Source: three-view drawing plus pictorial views. Frame: mm from the lowest corner of the part. Give positions to 0.01 mm unless a question says otherwise; leave off trailing zeros. Order: outer loops, then holes, each group sorted by start corner. A loop starts at its lowest first (then second) coordinate and runs counter-clockwise, first axis right, second up. Notation, with made-up numbers: (84.25, 56) - (120.25, 56) arc R23 ccw to (120.25, 79) - close; hole circle Ø10 at (39.5, 83). An arc over 180 degrees is marked (long way). Answer in a Markdown table with one row per item. Add a question column.
1. Ray query, line 1 (Z direction, x = 4, y = 61); line 2 (X direction, y = 32, z = 4.25). Return the intervals inside material, ascending. Write a range as [from, to].
2. Section query B-B on y = 40. Return loops of the section in (x, z).
3. Section query A-A on x = 4. Return loops of the section in (y, z), and give its area (3 significant figures).
4. Section query C-C on z = 1. Return loops of the section in (x, y).
5. Contact query for flat-ended pins moving along their axis: pin 1 (1.1 mm diameter, centred on y = 62, z = 7.5, fed in from -X); pin 2 (1 mm diameter, centred on x = 1.5, z = 5, fed in from -Y); pin 3 (0.8 mm diameter, centred on y = 2.5, z = 7.5, fed in from -X); pin 4 (0.8 mm diameter, centred on y = 3, z = 7.5, fed in from +X). Output: stop coordinate, or through.
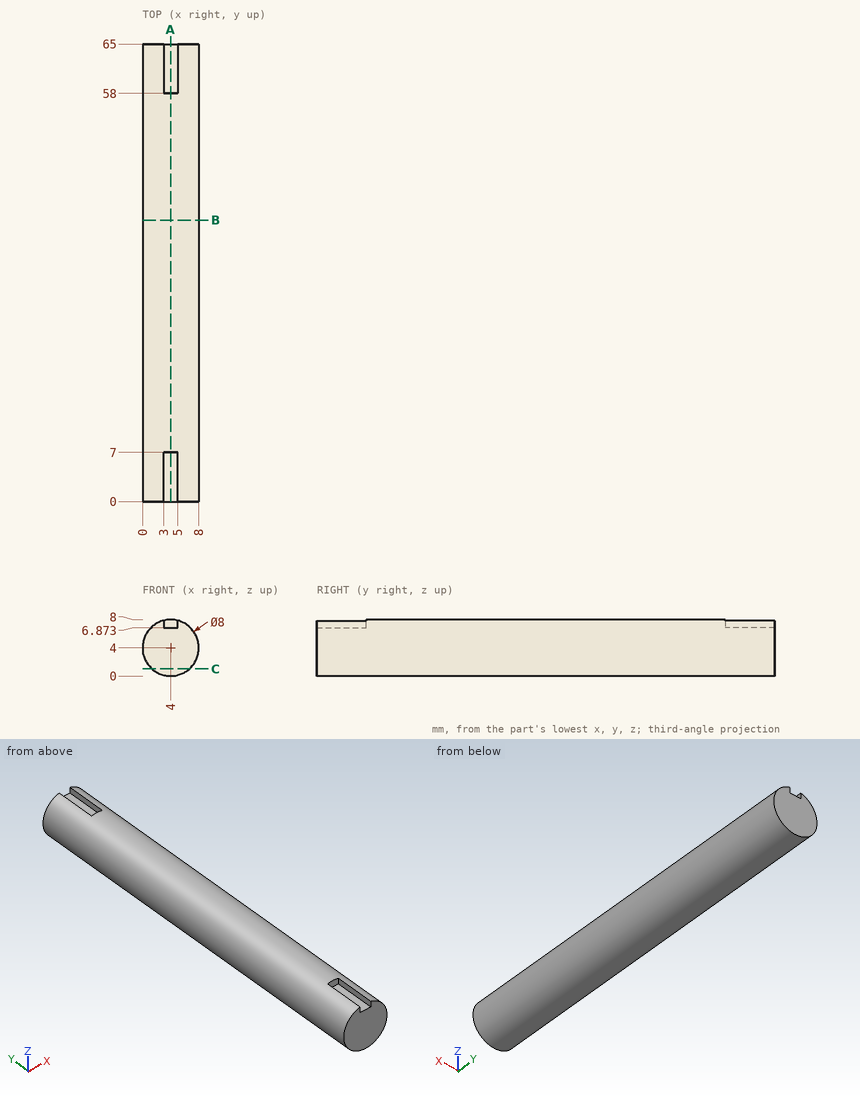
Answer:
| question | item | result |
|---|---|---|
| 1 | line 1 | z = [0, 6.87] |
| 1 | line 2 | x = [0.01, 7.99] |
| 2 | outline | circle Ø8 at (4, 4) |
| 3 | outline | (0, 0) - (65, 0) - (65, 6.87) - (58, 6.87) - (58, 8) - (7, 8) - (7, 6.87) - (0, 6.87) - close |
| 3 | area | 504 mm² |
| 4 | outline | (1.35, 0) - (6.65, 0) - (6.65, 65) - (1.35, 65) - close |
| 5 | pin 1 | stops at x = 1.3 |
| 5 | pin 2 | stops at y = 0 |
| 5 | pin 3 | stops at x = 1.47 |
| 5 | pin 4 | stops at x = 6.53 |
